Here's the drawing with two shaded views (mm, measured from the low corner). I have some questions. A direction names the side the tool comes from. Round coordinates to 2 decimals unless told otherwise and drop trailing zeros. Loops run counter-clockwise (first coordinate to the right, second up) from the corner with the lowest first, then second, coordinate; pieces in that order, holes last. Notation, with made-up numbers: (37.5, -36) -> (73.5, -36) arc R20 ccw to (73.5, -14) -> close; hole circle Ø2 at (-7.75, 82.25). An arc over 180 degrees is marked (long way). Write each question's results on one line, items separated by ' | '. Start each with the question number.
1) For P1, Ø2, axis at x = 8, z = 8, coming from the +Y side; P2, Ø1.5, axis at x = 4, z = 9.5, coming from the +Y side; P3, Ø5, axis at x = 12, y = 2, coming from the -Z side; P4, Ø1, axis at y = 9, z = 1, coming from the -X side, each with a flat end and sliding along its axis, tell me the tip position at first contact or that it passes through.
2) If I drill on probe 1 along Z at (x, y) = (7.25, 11.5); probe 2 along Z at (x, y) = (2.75, 7); probe 3 along X at (y, z) = (4.75, 7.5), over which ranges is the centre line in solid material (lowest first)?
3) Imagine slicing it at C-C, the plane z = 10.75. List the corners of the cut face in (x, y) for me, plus the area to 3 significant figures.
4) Which directions (+Z, -Z, +X, -X, +Y, -Y) give clear straight access to the entire face, cutting with the end or side of a thin tool? Please do the marked faces 1 and 2.
5) Imagine slicing it at B-B, the plane x = 7. List the corners of the cut face in (y, z) for me.
6) Imagine slicing it at D-D, the plane y = 10.25. List the corners of the cut face in (x, z) for me, plus the area to 3 significant figures.
7) Imagine slicing it at A-A, the plane y = 7. List the corners of the cut face in (x, z) for me.
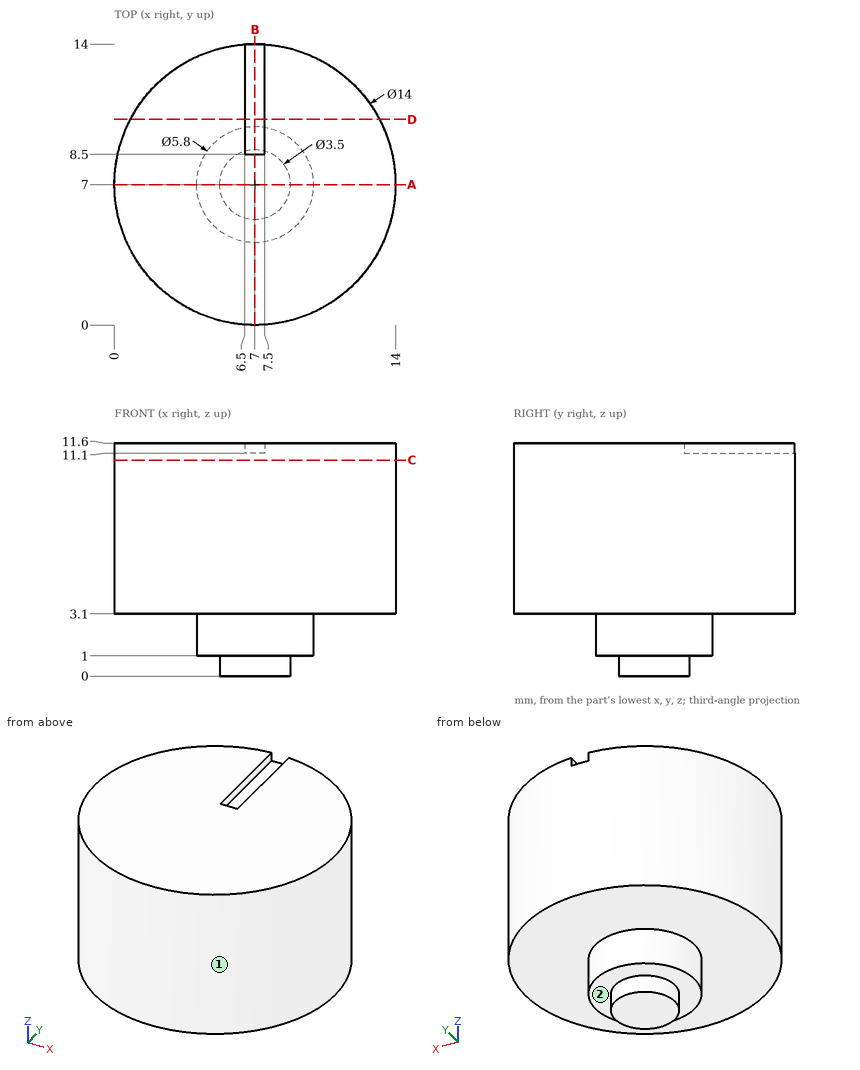
Checked values:
1) P1: y = 14 | P2: y = 13.63 | P3: z = 3.1 | P4: x = 4.52
2) probe 1: 3.1 to 11.1 | probe 2: 3.1 to 11.6 | probe 3: 0.37 to 13.63
3) outline: circle Ø14 at (7, 7) | area: 154 mm^2
4) face 1: +Z, -Z | face 2: -Z
5) outline: (0, 3.1) -> (4.1, 3.1) -> (4.1, 1) -> (5.25, 1) -> (5.25, 0) -> (8.75, 0) -> (8.75, 1) -> (9.9, 1) -> (9.9, 3.1) -> (14, 3.1) -> (14, 11.1) -> (8.5, 11.1) -> (8.5, 11.6) -> (0, 11.6) -> close
6) outline: (0.8, 3.1) -> (13.2, 3.1) -> (13.2, 11.6) -> (7.5, 11.6) -> (7.5, 11.1) -> (6.5, 11.1) -> (6.5, 11.6) -> (0.8, 11.6) -> close | area: 105 mm^2
7) outline: (0, 3.1) -> (4.1, 3.1) -> (4.1, 1) -> (5.25, 1) -> (5.25, 0) -> (8.75, 0) -> (8.75, 1) -> (9.9, 1) -> (9.9, 3.1) -> (14, 3.1) -> (14, 11.6) -> (0, 11.6) -> close
